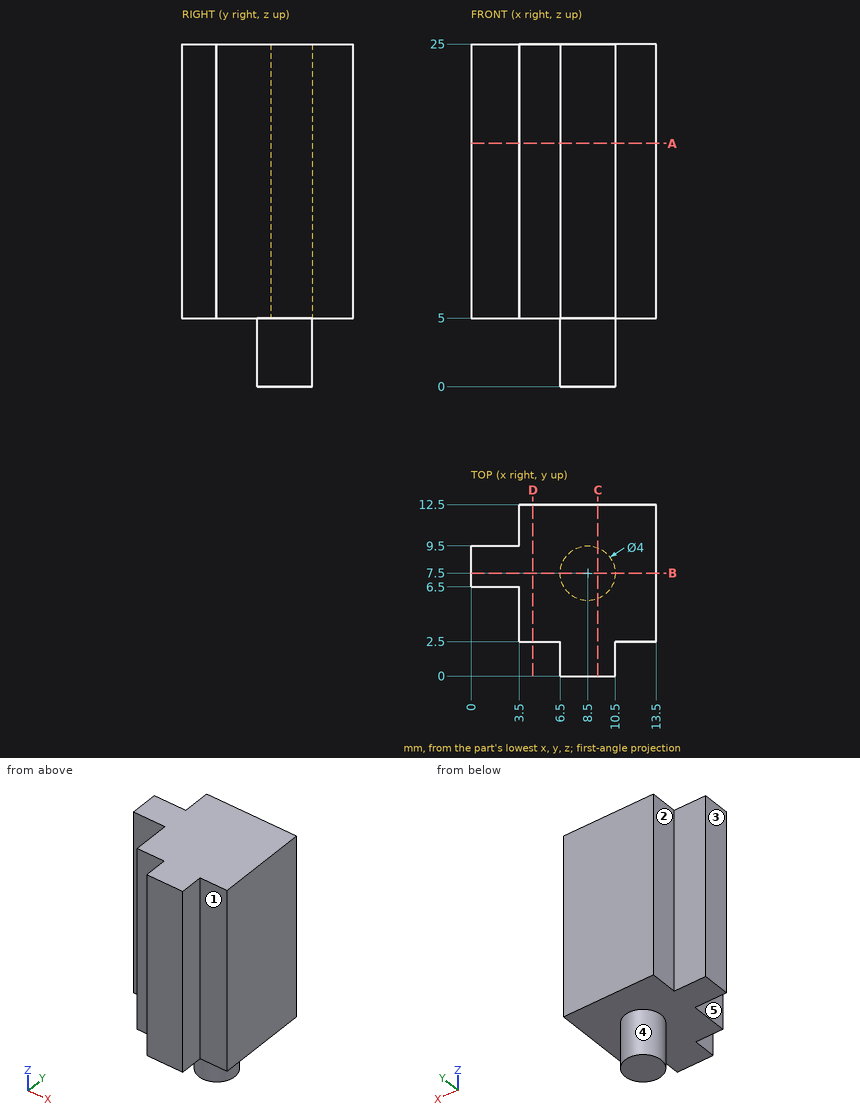
Geometry check sheet. Reference: drawing and pictorial views, mm from the part's lowest x, y, z. A direction names the side the tool comes from. Give positions to 0.01 mm unless a question says otherwise; leave off trailing zeros. Order: outer loops, then holes, each group sorted by start corner. A loop starts at its lowest first (then second) coordinate and runs counter-clockwise, first axis right, second up.
1. Section check B-B, the plane y = 7.5. Enter the section's corners in (x, z).
2. Section check C-C, the plane x = 9.25. Enter the section's corners in (y, z).
3. Gauge pin test, flat ends, axial feed: pin 1 Ø1 at (x, z) = (2.5, 13.5) entering from -Y; pin 2 Ø0.9 at (x, z) = (4.5, 18) entering from -Y; pin 3 Ø2.5 at (y, z) = (11.5, 12.5) entering from -X. Record the tip position at first contact, or that the pin passes through.
4. Section check A-A, the plane z = 17.75. Enter the section's corners in (x, y).
5. Section check D-D, the plane x = 4.5. Enter the section's corners in (y, z), and give its area (3 significant figures).
6. Thickness scan on L1, parallel to Z at x = 2.75, y = 7.5; L2, parallel to X at y = 5.25, z = 19; L3, parallel to X at y = 1, z = 16. Record the ranges inside material, lowest first.
7. Access from +Z, -Z, +X, -X, +Y, -Y to the whole of each face (thin tool, end or side, straight path). Record for the marked faces 1, 2, 3, 4 and 5.
Values follow:
1. outline: (0, 5) - (6.5, 5) - (6.5, 0) - (10.5, 0) - (10.5, 5) - (13.5, 5) - (13.5, 25) - (0, 25) - close
2. outline: (0, 5) - (5.65, 5) - (5.65, 0) - (9.35, 0) - (9.35, 5) - (12.5, 5) - (12.5, 25) - (0, 25) - close
3. pin 1: stops at y = 6.5
3. pin 2: stops at y = 2.5
3. pin 3: stops at x = 3.5
4. outline: (0, 6.5) - (3.5, 6.5) - (3.5, 2.5) - (6.5, 2.5) - (6.5, 0) - (10.5, 0) - (10.5, 2.5) - (13.5, 2.5) - (13.5, 12.5) - (3.5, 12.5) - (3.5, 9.5) - (0, 9.5) - close
5. outline: (2.5, 5) - (12.5, 5) - (12.5, 25) - (2.5, 25) - close
5. area: 200 mm2
6. L1: z = 5 to 25
6. L2: x = 3.5 to 13.5
6. L3: x = 6.5 to 10.5
7. face 1: +Z, -Z, +X, -Y
7. face 2: +Z, -Z, -X, +Y
7. face 3: +Z, -Z, -X, +Y, -Y
7. face 4: -Z
7. face 5: +Z, -Z, -X, -Y
